Source: CAD feature listing. Evaluate the final solid. Frame: model axes, mm. A direction names the side the tool comes from. Give positions to 0.01 mm unless a question says otherwise; leave off trailing zeros. Order: outer loops, then holes, each group sorted by start corner. A loop starts at its lowest first (then second) coordinate and runs counter-clockwise, first axis right, second up.
Autodesk Inventor part; units mm, degrees
ref_plane "YZ Plane" through (0, 0, 0) normal (1, 0, 0) x (0, 1, 0)
ref_plane "XZ Plane" through (0, 0, 0) normal (0, 1, 0) x (-1, 0, 0)
ref_plane "XY Plane" through (0, 0, 0) normal (0, 0, 1) x (1, 0, 0)
sketch "スケッチ1" plane through (0, 0, 0) normal (0, 0, 1) x (1, 0, 0)
  circle A0 centre (21.005288, 4.842186) radius 2
  circle A1 centre (0, 0) radius 2
  circle A2 centre (81.171801, -23.481667) radius 63
  arc A3 (-1.921226, 0.555779) -> (4.088443, -62.729672) centre (81.171801, -23.481667) ccw
  line L0 (0, 2) -> (9.827028, 2)
  line L1 (11.368602, 2.725814) -> (16.319283, 8.715397)
  line L2 (19.135043, 8.982785) -> (33.924305, -3.241258)
  line L3 (8.206239, 4.393532) -> (1.777293, 9.707368)
  line L4 (40.328272, 40.117124) -> (11.021999, 4.660921)
  arc A4 (9.827028, 2) -> (11.368602, 2.725814) centre (9.827028, 4) ccw
  arc A5 (19.135043, 8.982785) -> (16.319283, 8.715397) centre (17.860857, 7.441211) ccw
  arc A6 (34.516338, -5.502018) -> (38.734488, -49.921682) centre (81.171801, -23.481667) ccw
  circle A7 centre (5.870717, -61.822204) radius 2
  circle A8 centre (27.411976, -62.624114) radius 2
  line L5 (81.171801, -23.481667) -> (18.171801, -23.481667) construction
  line L6 (38.578569, -52.253469) -> (26.354526, -67.042731)
  line L7 (17.573011, -64.325196) -> (53.029214, -93.631469)
  line L8 (17.573011, -64.325196) -> (53.029214, -93.631469)
  line L9 (9.443415, -71.02153) -> (14.757251, -64.592584)
  line L10 (23.538766, -67.310119) -> (17.549183, -62.359438)
  arc A9 (23.538766, -67.310119) -> (26.354526, -67.042731) centre (24.812952, -65.768545) ccw
  line L11 (15.898547, -61.93676) -> (6.247168, -63.786456)
  arc A10 (17.549183, -62.359438) -> (15.898547, -61.93676) centre (16.274997, -63.901012) ccw
  arc A11 (34.516338, -5.502018) -> (33.924305, -3.241258) centre (32.65012, -4.782832) ccw
  arc A12 (38.578569, -52.253469) -> (38.734488, -49.921682) centre (37.036995, -50.979283) ccw
  circle A13 centre (5.870717, -61.822204) radius 1
  circle A14 centre (27.411976, -62.624114) radius 1
  circle A15 centre (21.005288, 4.842186) radius 1
  circle A16 centre (0, 0) radius 1
  line L12 (0, 0) -> (5.870717, -61.822204) construction
  line L13 (32.285214, -12.988736) -> (35.134053, -42.988736)
  point P0 (0, 0)
  point P1 (35.050768, -4.172335)
  point P2 (39.509645, -51.127006)
  dimension "d0" = 1.5
  dimension "d1" = 2
  dimension "d3" = 50
  dimension "d8" = 2
  dimension "d9" = 2
  dimension "d12" = 30
extrude "押し出し1" add sketch "スケッチ1" along normal blind 1.6 contours A0 | A8 | L2 A2 L6 A9 L10 A10 L11 A7 A3 A1 L0 A4 L1 A5 | L2 A11 A6 A12 L6 A2 | L13 A6 | A1 | A7
fillet "フィレット1" radius 2 2 edges at (35.1341, -42.9887, 0.8) (32.2852, -12.9887, 0.8)
properties part number "MainMCU_PCB"
1) Ray query, L1, parallel to Y at x = 18, z = 1.35; L2, parallel to Y at x = 6.5, z = 0.5; L3, parallel to Y at x = 31.5, z = 1.35. Return the intervals inside material, ascending.
Checks:
L1: y = -62.73 to 9.44
L2: y = -63.74 to -62.6, -61.05 to 2
L3: y = -60.82 to -1.24
2) Section query B-B on z = 1. Output: boundary loops of the cut face in (x, y) (3 decimals).
Checks:
outline: (-1.921, 0.556) arc R86.5 ccw to (4.088, -62.73) arc R2 ccw to (6.247, -63.786) - (15.899, -61.937) arc R2 cw to (17.549, -62.359) - (23.539, -67.31) arc R2 ccw to (26.355, -67.043) - (38.579, -52.253) arc R2 ccw to (38.734, -49.922) arc R50 cw to (35.259, -43.281) arc R2 cw to (35.105, -42.678) - (32.315, -13.299) arc R2 cw to (32.353, -12.678) arc R50 cw to (34.516, -5.502) arc R2 ccw to (33.924, -3.241) - (19.135, 8.983) arc R2 ccw to (16.319, 8.715) - (11.369, 2.726) arc R2 cw to (9.827, 2) - (0, 2) arc R2 ccw to start; hole circle Ø2 at (0, 0); hole circle Ø2 at (5.871, -61.822); hole circle Ø2 at (21.005, 4.842); hole circle Ø2 at (27.412, -62.624)
3) Section query C-C on y = -56. Output: boundary loops of the cut face in (x, z).
Checks:
outline: (1.02, 0) - (35.48, 0) - (35.48, 1.6) - (1.02, 1.6) - close
4) First-contact query: pin 1 Ø0.5 at (x, z) = (4.5, 0.5) entering from +Y. Flat tip, straight axial feed; report the tip coordinate or a pass-through.
Checks:
pin 1: stops at y = 2
5) Pull-direction query (Y, two-part tool) for faces 5 (the face through (5.654, -60.846, 0.789)), 6 (the face through (17, -29, 1.6)), 7 (the face through (26.426, 2.956, 0.789)); classes: +Y half, -Y half, draft (parallel to the pull), parting line (faces both ways), or undercut.
Checks:
face 5: undercut
face 6: draft
face 7: +Y half
6) Section query A-A on x = 21. Output: boundary loops of the cut face in (y, z), and give its area (3 significant figures).
Checks:
outline: (-65.21, 0) - (3.84, 0) - (3.84, 1.6) - (-65.21, 1.6) - close; (5.84, 0) - (7.44, 0) - (7.44, 1.6) - (5.84, 1.6) - close
area: 113 mm2
7) Reachability of faces 1 (the face through (33.69, -27.78, 0.79)), 2 (the face through (36.897, -46.713, 0.789)), 3 (the face through (5, 2, 1)), 4 (the face through (20.586, -64.869, 0.789)) from +Z, -Z, +X, -X, +Y, -Y: full face, straight path, thin tool, end or side. Return the list, or none.
Checks:
face 1: +Z, -Z, +X
face 2: +Z, -Z, +X, +Y
face 3: +Z, -Z, -X, +Y
face 4: +Z, -Z, -Y
